Autodesk Inventor part; units mm, degrees
ref_plane "YZ Plane" through (0, 0, 0) normal (1, 0, 0) x (0, 1, 0)
ref_plane "XZ Plane" through (0, 0, 0) normal (0, 1, 0) x (-1, 0, 0)
ref_plane "XY Plane" through (0, 0, 0) normal (0, 0, 1) x (1, 0, 0)
sketch "Sketch1" plane through (0, 0, 0) normal (1, 0, 0) x (0, 1, 0)
  line L0 (0, 0) -> (25.4, 0)
  line L1 (3.2512, -25.4) -> (0, -25.4)
  line L2 (0, -25.4) -> (0, 0)
  line L3 (3.2512, -3.2512) -> (25.4, -3.2512)
  line L4 (3.2512, -25.4) -> (3.2512, -3.2512)
  line L5 (25.4, 0) -> (25.4, -3.2512)
  dimension "d0" = 25.4
  dimension "d1" = 3.2512
extrude "Extrusion1" add sketch "Sketch1" along normal blind 1828.8
sketch "Sketch2" plane through (0, 0, 0) normal (0, 0, 1) x (1, 0, 0)
  line L0 (0, 0) -> (0, 25.4)
  line L1 (0, 12.7) -> (44.4361, 12.7) construction
  circle A0 centre (12.7, 12.7) radius 3.175
  circle A1 centre (139.7, 12.7) radius 3.175
  dimension "d4" = 6.35
  dimension "d5" = 12.7
  dimension "d6" = 139.7
extrude "Extrusion2" cut sketch "Sketch2" against normal blind 1828.8
sketch "Sketch3" plane through (0, 0, -25.4) normal (0, -1, 0) x (1, 0, 0)
  line L0 (0, 0) -> (0, 25.4)
  line L1 (0, 12.7) -> (119.8367, 12.7) construction
  circle A0 centre (12.7, 12.7) radius 3.175
  circle A1 centre (139.7, 12.7) radius 3.175
  dimension "d9" = 6.35
  dimension "d10" = 12.7
  dimension "d11" = 139.7
extrude "Extrusion3" cut sketch "Sketch3" against normal blind 1828.8
properties part number "Upper Long L"
Work out the finished part from the listing and answer in its coordinate system (mm). Give positions to 0.01 mm unless a question says otherwise; leave off trailing zeros. Write each loop counter-clockwise with the first axis right and the second up, starting at its lowest first coordinate (ties: lowest second). Pieces come first, ordered by that corner, then holes.
Q1. Given pin 1 (10 mm diameter, centred on x = 1601, y = 13.5, fed in from -Z); pin 2 (10 mm diameter, centred on x = 139.7, z = -12.7, fed in from +Y), each flat-ended and moving along its own axis, determine where each tip first touches the part or whether it passes through.
Answer:
pin 1: stops at z = -3.25
pin 2: stops at y = 3.25
Q2. Straight lines are drawn through the part: L1, parallel to Y at x = 12.7, z = -2.6 (3 decimals); L2, parallel to Z at x = 139.7, y = 1.15 (3 decimals); L3, parallel to Z at x = 1609, y = 23. For each, find the intervals that lie inside material, in ascending order.
Answer:
L1: y = 0 to 9.525, 15.875 to 25.4
L2: z = -25.4 to -15.875, -9.525 to 0
L3: z = -3.25 to 0
Q3. The part is cut by section A-A on x = 1602.5. Give the vertices of the cut face in (y, z), and give its area (3 significant figures).
Answer:
outline: (0, -25.4) - (3.25, -25.4) - (3.25, -3.25) - (25.4, -3.25) - (25.4, 0) - (0, 0) - close
area: 155 mm2
